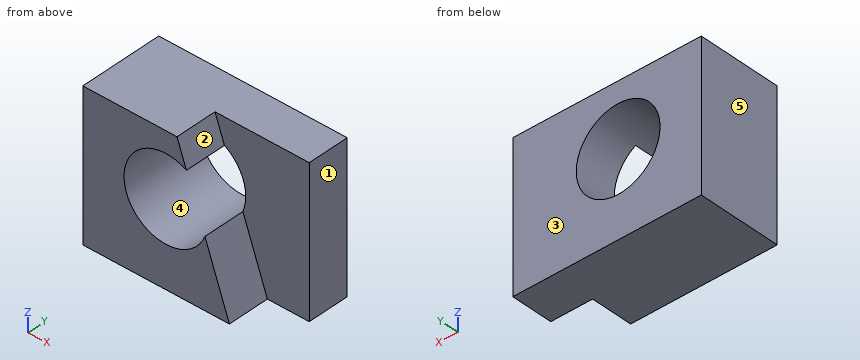
```python
from build123d import *

# Parameters (mm, degrees)
F0_W     = 57.15
F0_H     = 44.45
F1_DEPTH = 25.4
F2_R     = 12.7
F3_DEPTH = 25.401
F5_DEPTH = 12.7


with BuildPart() as f1:
    # F0 (on Front) → F1 (new body)
    with BuildSketch(Plane.XZ):
        with Locations((28.575, 22.225)):
            Rectangle(F0_W, F0_H)
    extrude(amount=F1_DEPTH)

    # F2 (on face) → F3 (cut, through all)
    with BuildSketch(Plane.XZ.offset(25.4)):
        with Locations((25.2007812379, 25.4)):
            Circle(F2_R)
    extrude(amount=-F3_DEPTH, mode=Mode.SUBTRACT)

    # F4 (on face) → F5 (cut)
    with BuildSketch(Plane.XZ.offset(25.4)):
        with BuildLine():
            Line((57.15, 44.45), (28.575, 44.45))
            Line((28.575, 44.45), (31.4249152112, 36.4702374086))
            ThreePointArc((31.4249152112, 36.4702374086), (36.1629092581, 31.8126242108), (37.9007812379, 25.4))
            ThreePointArc((37.9007812379, 25.4), (37.6810755571, 23.0479256591), (37.029560182, 20.7772314905))
            Line((37.029560182, 20.7772314905), (44.45, 0))
            Line((44.45, 0), (57.15, 0))
            Line((57.15, 0), (57.15, 44.45))
        make_face()
    extrude(amount=-F5_DEPTH, mode=Mode.SUBTRACT)


solid = f1.part
```
The listing builds one solid part. Answer for the finished solid, in the listing's coordinates (mm). Face numbers are marked on the shaded views. A direction names the side the tool comes from. Coordinates: 2 decimals unless noted, no trailing zeros. Write each loop counter-clockwise with the first axis right and the second up, starting at its lowest first coordinate (ties: lowest second). Pieces come first, ordered by that corner, then holes. Notation, with made-up numbers: (-9.5, 39.5) - (46.5, 39.5) arc R7 ccw to (46.5, 49.5) - close; hole circle Ø10 at (55.5, 74.5). An arc over 180 degrees is marked (long way). One line per item, written item: value.
1) Find section A-A (z = 25.4). Give the vertices of the cut face in (x, y), and give its area (3 significant figures).
Geometry check:
outline: (0, -25.4) - (12.5, -25.4) - (12.5, 0) - (0, 0) - close; (37.9, -12.7) - (57.15, -12.7) - (57.15, 0) - (37.9, 0) - close
area: 562 mm2
2) A tool of negligible diameter and unlimited length cuts with its end or side. For the marked faces 1 and 2, from which of +Z, -Z, +X, -X, +Y, -Y can it reach the whole face along a straight path? Write none if from no direction.
Geometry check:
face 1: +Z, -Z, +X, +Y, -Y
face 2: +Z, +X, -Y
3) Consider line 1 along Z through (x, y) = (14, -5); line 2 along X through (y, z) = (-1.25, 19); line 3 along Z through (x, y) = (29, -1.5). Determine where each line is inside the solid, lowest interval first. Write a range as from..to.
Geometry check:
line 1: z = 0..19.41, 31.39..44.45
line 2: x = 0..14.23, 36.17..57.15
line 3: z = 0..13.28, 37.52..44.45
4) Find section C-C (x = 30). Give the vertices of the cut face in (y, z).
Geometry check:
outline: (-25.4, 0) - (0, 0) - (0, 13.64) - (-25.4, 13.64) - close; (-25.4, 37.16) - (0, 37.16) - (0, 44.45) - (-12.7, 44.45) - (-12.7, 40.46) - (-25.4, 40.46) - close
5) For a pull along X with two mould halves and no side action, classify the marked faces 3, 4 and 5 as pulls with the +X half, pulls with the -X half, needs draft (parallel to the pull), parting line crosses it, or undercut.
Geometry check:
face 3: needs draft
face 4: undercut
face 5: pulls with the -X half
6) Find section D-D (y = -16.75). Give the vertices of the cut face in (x, z) (3 decimals).
Geometry check:
outline: (0, 0) - (44.45, 0) - (37.03, 20.777) arc R12.7 cw (long way) to (31.425, 36.47) - (28.575, 44.45) - (0, 44.45) - close
7) Find section B-B (y = -3.5). Give the vertices of the cut face in (x, z).
Geometry check:
outline: (0, 0) - (57.15, 0) - (57.15, 44.45) - (0, 44.45) - close; hole circle Ø25.4 at (25.2, 25.4)
